```python
from build123d import *

# Parameters (mm, degrees)
SKETCH1_W                    = 275
SKETCH1_H                    = 33
BOSS_EXTRUDE1_DEPTH          = 12
CUT_EXTRUDE1_REACH           = 141.005
SKETCH2_R                    = 7
BOSS_EXTRUDE2_DEPTH          = 12
CUT_EXTRUDE2_REACH           = 250.863
SKETCH4_R                    = 2.5
CUT_EXTRUDE3_REACH           = 278.522
SKETCH5_W                    = 14
SKETCH5_H                    = 6
FILLET1_R                    = 2
FILLET1_OF_MIRROR2_R         = 2
CHAMFER1_SIZE                = 10
CUT_EXTRUDE4_REACH           = 278.522
SKETCH6_W                    = 12
SKETCH6_H                    = 30
CHAMFER2_SIZE                = 10
F_6_0_6_DIAMETER_HOLE1_D     = 6
F_6_0_6_DIAMETER_HOLE2_D     = 6
F_6_0_6_DIAMETER_HOLE2_DEPTH = 12
F_6_0_6_DIAMETER_HOLE2_TIP   = 1.802581857


with BuildPart() as part:
    # Sketch1 → Boss-Extrude1 (new body)
    with BuildSketch(Plane.XY):
        Rectangle(SKETCH1_W, SKETCH1_H)
    extrude(amount=BOSS_EXTRUDE1_DEPTH)

    # Sketch2 → Cut-Extrude1 (cut, up to next)
    with BuildSketch(Plane.XY.offset(12), mode=Mode.PRIVATE) as cut_extrude1_sk1:
        with Locations((0, 1)):
            Circle(SKETCH2_R)
    cut_extrude1_tool1 = extrude(cut_extrude1_sk1.sketch, amount=-CUT_EXTRUDE1_REACH, mode=Mode.PRIVATE) & part.part
    add(cut_extrude1_tool1.solids().sort_by_distance((0, 1, 12))[0], mode=Mode.SUBTRACT)

    # Sketch3 → Boss-Extrude2 (add)
    with BuildSketch(Plane.XY.offset(12)):
        Polygon((-210, 16.5), (210, 16.5), (210, 179.5), (183, 179.5), (183, 46.5), (-183, 46.5), (-183, 179.5), (-210, 179.5), align=None)
    extrude(amount=-BOSS_EXTRUDE2_DEPTH)

    # Sketch4 → Cut-Extrude2 (cut, up to next)
    with BuildSketch(Plane(origin=(0, 46.5, 0), x_dir=(1, 0, 0), z_dir=(0, 1, 0)), mode=Mode.PRIVATE) as cut_extrude2_sk1:
        with Locations(Location((-144, -6, 0), (0, 0, 270))):
            Circle(SKETCH4_R)
    cut_extrude2_tool1 = extrude(cut_extrude2_sk1.sketch, amount=-CUT_EXTRUDE2_REACH, mode=Mode.PRIVATE) & part.part
    # Sketch4 → Cut-Extrude2 (cut, up to next)
    with BuildSketch(Plane(origin=(0, 46.5, 0), x_dir=(1, 0, 0), z_dir=(0, 1, 0)), mode=Mode.PRIVATE) as cut_extrude2_sk2:
        with Locations(Location((-176, -6, 0), (0, 0, 270))):
            Circle(SKETCH4_R)
    cut_extrude2_tool2 = extrude(cut_extrude2_sk2.sketch, amount=-CUT_EXTRUDE2_REACH, mode=Mode.PRIVATE) & part.part
    cut_extrude2_1 = cut_extrude2_tool1.solids().sort_by_distance((-144, 46.5, 6))[0]
    add(cut_extrude2_1, mode=Mode.SUBTRACT)
    cut_extrude2_2 = cut_extrude2_tool2.solids().sort_by_distance((-176, 46.5, 6))[0]
    add(cut_extrude2_2, mode=Mode.SUBTRACT)
    cut_extrude2 = cut_extrude2_1 + cut_extrude2_2  # Cut-Extrude2 as one shape, for the pattern or mirror that repeats it

    # Mirror1: Cut-Extrude2 across plane
    add(cut_extrude2.mirror(Plane(origin=(0, 0, 0), x_dir=(0, 0, 1), z_dir=(1, 0, 0))), mode=Mode.SUBTRACT)

    # Sketch5 → Cut-Extrude3 (cut, up to next)
    with BuildSketch(Plane.XY.offset(12), mode=Mode.PRIVATE) as cut_extrude3_sk1:
        with Locations((-176, 43.5)):
            Rectangle(SKETCH5_W, SKETCH5_H)
    cut_extrude3_tool1 = extrude(cut_extrude3_sk1.sketch, amount=-CUT_EXTRUDE3_REACH, mode=Mode.PRIVATE) & part.part
    # Sketch5 → Cut-Extrude3 (cut, up to next)
    with BuildSketch(Plane.XY.offset(12), mode=Mode.PRIVATE) as cut_extrude3_sk2:
        with Locations((-144, 43.5)):
            Rectangle(SKETCH5_W, SKETCH5_H)
    cut_extrude3_tool2 = extrude(cut_extrude3_sk2.sketch, amount=-CUT_EXTRUDE3_REACH, mode=Mode.PRIVATE) & part.part
    cut_extrude3_1 = cut_extrude3_tool1.solids().sort_by_distance((-176, 43.5, 12))[0]
    add(cut_extrude3_1, mode=Mode.SUBTRACT)
    cut_extrude3_2 = cut_extrude3_tool2.solids().sort_by_distance((-144, 43.5, 12))[0]
    add(cut_extrude3_2, mode=Mode.SUBTRACT)
    cut_extrude3 = cut_extrude3_1 + cut_extrude3_2  # Cut-Extrude3 as one shape, for the pattern or mirror that repeats it

    # Fillet1
    fillet1_edges = [part.edges().sort_by_distance(p)[0] for p in [
        (-169, 40.5, 6),
        (-183, 40.5, 6),
        (-137, 40.5, 6),
        (-151, 40.5, 6),
    ]]
    fillet(fillet1_edges, radius=FILLET1_R)

    # Mirror2: Cut-Extrude3 across plane
    add(cut_extrude3.mirror(Plane(origin=(0, 0, 0), x_dir=(0, 0, 1), z_dir=(1, 0, 0))), mode=Mode.SUBTRACT)

    # Fillet1 of Mirror2
    fillet1_of_mirror2_edges = [part.edges().sort_by_distance(p)[0] for p in [
        (169, 40.5, 6),
        (183, 40.5, 6),
        (137, 40.5, 6),
        (151, 40.5, 6),
    ]]
    fillet(fillet1_of_mirror2_edges, radius=FILLET1_OF_MIRROR2_R)

    # Chamfer1
    chamfer1_edges = [part.edges().sort_by_distance(p)[0] for p in [
        (210, 16.5, 6),
        (-210, 16.5, 6),
    ]]
    chamfer(chamfer1_edges, length=CHAMFER1_SIZE)

    # Sketch6 → Cut-Extrude4 (cut, up to next)
    with BuildSketch(Plane.XY.offset(12), mode=Mode.PRIVATE) as cut_extrude4_sk1:
        with Locations((-194, 164.5)):
            Rectangle(SKETCH6_W, SKETCH6_H)
    cut_extrude4_tool1 = extrude(cut_extrude4_sk1.sketch, amount=-CUT_EXTRUDE4_REACH, mode=Mode.PRIVATE) & part.part
    cut_extrude4 = cut_extrude4_tool1.solids().sort_by_distance((-194, 164.5, 12))[0]
    add(cut_extrude4, mode=Mode.SUBTRACT)

    # Mirror3: Cut-Extrude4 across plane
    add(cut_extrude4.mirror(Plane(origin=(0, 0, 0), x_dir=(0, 0, 1), z_dir=(1, 0, 0))), mode=Mode.SUBTRACT)

    # Chamfer2
    chamfer2_edges = [part.edges().sort_by_distance(p)[0] for p in [
        (210, 179.5, 6),
        (-210, 179.5, 6),
    ]]
    chamfer(chamfer2_edges, length=CHAMFER2_SIZE - 0.0001)  # a hair under: the kernel refuses the full size

    # Ø6.0 (6) Diameter Hole1 (through all)
    with Locations(Plane.XY.offset(12)):
        with Locations((-195, 40.5), (-195, 131.5)):
            f_6_0_6_diameter_hole1 = Hole(F_6_0_6_DIAMETER_HOLE1_D / 2)

    # Mirror4: Ø6.0 (6) Diameter Hole1 across plane
    add(f_6_0_6_diameter_hole1.mirror(Plane(origin=(0, 0, 0), x_dir=(0, 0, 1), z_dir=(1, 0, 0))), mode=Mode.SUBTRACT)

    # Ø6.0 (6) Diameter Hole2
    with Locations(Plane.XY.offset(12)):
        with Locations((-97.5, 13.5), (-40, 13.5), (40, 13.5), (97.5, 13.5)):
            Hole(F_6_0_6_DIAMETER_HOLE2_D / 2, depth=F_6_0_6_DIAMETER_HOLE2_DEPTH)
            with Locations((0, 0, -(F_6_0_6_DIAMETER_HOLE2_DEPTH + F_6_0_6_DIAMETER_HOLE2_TIP / 2))):  # 118° drill point
                Cone(0, F_6_0_6_DIAMETER_HOLE2_D / 2, F_6_0_6_DIAMETER_HOLE2_TIP, mode=Mode.SUBTRACT)


solid = part.part
```
Part model, mm, in its own coordinate system. A direction names the side the tool comes from. Round coordinates to 2 decimals unless told otherwise and drop trailing zeros. Loops run counter-clockwise (first coordinate to the right, second up) from the corner with the lowest first, then second, coordinate; pieces in that order, holes last. Notation, with made-up numbers: (-23.5, 25.5) -> (32.5, 25.5) arc R17 ccw to (32.5, 48.5) -> close; hole circle Ø9 at (67, -15.5). An arc over 180 degrees is marked (long way). Use one line per item in the form item = value. Start each with the question number.
Item 1: Band-saw the part on B-B (z = 6). Give the number of separate pieces and of enclosed holes in the cut face, plus the area to 3 significant figures.
Item 2: Band-saw the part on C-C (x = 87). List the corners of the cut face in (y, z).
Item 3: Two-plate mould, pull along X, no slides. Class faces 4 (the flat face through (-205.1, 21.6, 6.1)), 5 (the flat face through (137.5, 0, 6)), 6 (the flat face through (160, 46.5, 6)), 7 (the flat face through (-2, -16.5, 6)): released by +X, released by -X, zero draft, split by the parting line, or undercut.
Item 4: Drop flat-ended pins along their axis: pin 1 Ø3.5 at (x, y) = (-195, 40.5) entering from -Z; pin 2 Ø6 at (x, z) = (144, 6) entering from -Y; pin 3 Ø5 at (x, z) = (-140.5, 6) entering from +Y; pin 4 Ø6 at (x, z) = (-110.5, 4.5) entering from +Y. Give the stop position or say it passes through.
Item 5: Tool access for faces 1 (the flat face through (-169, 16.5, 6)), 2 (the flat face through (146.3, 40.5, 7.4)), 3 (the flat face through (168, 16.5, 6)): list every direction of +Z, -Z, +X, -X, +Y, -Y with a clear straight run to the whole face (end or side of a thin tool).
Item 6: Band-saw the part on A-A (y = 139). List the corners of the cut face in (x, z), plus the area to 3 significant figures.
Item 7: Drill centre lines: line 1 along Y through (x, z) = (-195, 8.75); line 2 along Z through (x, y) = (144, 26); line 3 along X through (y, z) = (52.5, 5.75). Where is each one in solid material? Low to high.
Data:
q1.separate_pieces = 5
q1.enclosed_holes = 9
q1.area = 26,700 mm^2
q2.outline = (-16.5, 0) -> (46.5, 0) -> (46.5, 12) -> (-16.5, 12) -> close
q3.face_4 = released by -X
q3.face_5 = released by +X
q3.face_6 = undercut
q3.face_7 = zero draft
q4.pin_1 = through
q4.pin_2 = 16.5
q4.pin_3 = 40.77
q4.pin_4 = 46.5
q5.face_1 = +Z, -Z, -X, -Y
q5.face_2 = +Z, -Z, +Y
q5.face_3 = +Z, -Z, +X, -Y
q6.outline = (-210, 0) -> (-183, 0) -> (-183, 12) -> (-210, 12) -> close; (183, 0) -> (210, 0) -> (210, 12) -> (183, 12) -> close
q6.area = 648 mm^2
q7.line_1 = 16.5 to 37.5, 43.5 to 128.5, 134.5 to 149.5
q7.line_2 = 0 to 3.5, 8.5 to 12
q7.line_3 = -210 to -183, 183 to 210
